Source: CAD feature listing. Evaluate the final solid. Frame: model axes, mm. A direction names the side the tool comes from. Coordinates: 2 decimals unless noted, no trailing zeros. Order: outer loops, then holes, each group sorted by start corner. A loop starts at its lowest first (then second) coordinate and runs counter-clockwise, first axis right, second up. Notation, with made-up numbers: (-37, 9.25) -> (21, 9.25) arc R34 cw to (21, 42.25) -> close; hole circle Ø8 at (6.25, 82.5). An arc over 180 degrees is marked (long way). Write item = value, one per line. Start each with the question number.
Item 1: Mould query, pull axis Z, two halves, no side actions, for faces 1 (the flat face through (-3.686, 11, 1)), 2 (the flat face through (27.7, -6.5, 36.367)), 3 (the flat face through (27, 10, 37)), 4 (the flat face through (-40, 10.642, 19)). Classes: released by +Z, released by -Z, zero draft, split by the parting line, or undercut.
Item 2: Ray query, line 1 along Y through (x, z) = (-41, 3); line 2 along Z through (x, y) = (-22, 14). Return the intervals inside material, ascending. Write a range as [from, to].
Item 3: Section query D-D (x = -39.5). Output: boundary loops of the cut face in (y, z).
Item 4: Section query B-B (z = 4.5). Output: boundary loops of the cut face in (x, y).
Item 5: Contact query for flat-ended pins moving along their axis: pin 1 (8 mm diameter, centred on x = -34.5, z = 12.5, fed in from -Y); pin 2 (1 mm diameter, centred on x = 28.5, z = 15.5, fed in from +Y); pin 3 (7.5 mm diameter, centred on y = -8.5, z = 12, fed in from -X). Output: stop coordinate, or through.
Item 6: Set-up query: faces 5 (the flat face through (29.47, -12, 20)), 6 (the flat face through (-38.216, -12, 20)), 7 (the flat face through (-41.716, 12, 20)), 8 (the flat face through (11, -13.208, 1)). Return all of +Z, -Z, +X, -X, +Y, -Y with unobstructed straight access to the full face (end or side cutting, diameter ignored); none if empty.
Item 7: Section query A-A (y = 0). Output: boundary loops of the cut face in (x, z).
Item 8: Section query C-C (x = 8). Output: boundary loops of the cut face in (y, z), then the cut area to 3 significant figures.
```python
from build123d import *

# Parameters (mm, degrees)
SKETCH1_W           = 105.78
SKETCH1_H           = 30
BOSS_EXTRUDE1_DEPTH = 2
SKETCH5_W           = 3.5
SKETCH5_H           = 2
BOSS_EXTRUDE2_DEPTH = 35
SKETCH6_W           = 3.5
SKETCH6_H           = 2
BOSS_EXTRUDE3_DEPTH = 35
SKETCH7_W           = 3.5
SKETCH7_H           = 0.495515405
BOSS_EXTRUDE4_DEPTH = 5
SKETCH9_W           = 3.5
SKETCH9_H           = 0.633233513
BOSS_EXTRUDE5_DEPTH = 5
SKETCH10_R          = 1.510168907
CUT_EXTRUDE2_DEPTH  = 72
SKETCH11_R          = 1.533572267
CUT_EXTRUDE3_DEPTH  = 42
SKETCH12_R          = 3.25
CUT_EXTRUDE4_DEPTH  = 15
FILLET1_R           = 0.8
SKETCH13_W          = 28.000104313
SKETCH13_H          = 4
CUT_EXTRUDE5_DEPTH  = 10


with BuildPart() as part:
    # Sketch1 → Boss-Extrude1 (new body)
    with BuildSketch(Plane.XY):
        Rectangle(SKETCH1_W, SKETCH1_H)
    extrude(amount=BOSS_EXTRUDE1_DEPTH)

    # Sketch5 → Boss-Extrude2 (add)
    with BuildSketch(Plane.XY.offset(2)):
        with Locations((27.719609025, 11.641851008)):
            Rectangle(SKETCH5_W, SKETCH5_H)
    boss_extrude2 = extrude(amount=BOSS_EXTRUDE2_DEPTH)

    # Sketch6 → Boss-Extrude3 (add)
    with BuildSketch(Plane.XY.offset(2)):
        with Locations((-39.966011677, 11.641851008)):
            Rectangle(SKETCH6_W, SKETCH6_H)
    boss_extrude3 = extrude(amount=BOSS_EXTRUDE3_DEPTH)

    # Sketch7 → Boss-Extrude4 (add)
    with BuildSketch(Plane.XZ.offset(-10.641851008)):
        with Locations((-39.966011677, 36.752242298)):
            Rectangle(SKETCH7_W, SKETCH7_H)
    boss_extrude4 = extrude(amount=BOSS_EXTRUDE4_DEPTH)

    # Sketch9 → Boss-Extrude5 (add)
    with BuildSketch(Plane.XZ.offset(-10.641851008)):
        with Locations((27.719609025, 36.683383244)):
            Rectangle(SKETCH9_W, SKETCH9_H)
    boss_extrude5 = extrude(amount=BOSS_EXTRUDE5_DEPTH)

    # Sketch10 → Cut-Extrude2 (cut)
    with BuildSketch(Plane.XY.offset(2)):
        with Locations(Location((27.719609025, 8.420134131, 0), (0, 0, 180))):
            Circle(SKETCH10_R)
    cut_extrude2 = extrude(amount=CUT_EXTRUDE2_DEPTH, mode=Mode.SUBTRACT)

    # Sketch11 → Cut-Extrude3 (cut)
    with BuildSketch(Plane.XY.offset(2)):
        with Locations(Location((-39.966011677, 8.661839338, 0), (0, 0, 180))):
            Circle(SKETCH11_R)
    cut_extrude3 = extrude(amount=CUT_EXTRUDE3_DEPTH, mode=Mode.SUBTRACT)

    # Mirror2: Boss-Extrude2, Boss-Extrude3, Boss-Extrude4, Boss-Extrude5, Cut-Extrude2, Cut-Extrude3 across plane
    add(boss_extrude2.mirror(Plane.ZX))
    add(boss_extrude3.mirror(Plane.ZX))
    add(boss_extrude4.mirror(Plane.ZX))
    add(boss_extrude5.mirror(Plane.ZX))
    add(cut_extrude2.mirror(Plane.ZX), mode=Mode.SUBTRACT)
    add(cut_extrude3.mirror(Plane.ZX), mode=Mode.SUBTRACT)

    # Sketch12 → Cut-Extrude4 (cut)
    with BuildSketch(Plane.XY.offset(2)):
        with Locations((-34.920285351, 0)):
            Circle(SKETCH12_R)
    extrude(amount=-CUT_EXTRUDE4_DEPTH, mode=Mode.SUBTRACT)

    # Fillet1
    fillet1_edges = [part.edges().sort_by_distance(p)[0] for p in [
        (29.469609025, 11.641851008, 2),
        (27.719609025, 12.641851008, 2),
        (25.969609025, 11.641851008, 2),
        (27.719609025, 10.641851008, 2),
        (-38.216011677, 11.641851008, 2),
        (-39.966011677, 12.641851008, 2),
        (-41.716011677, 11.641851008, 2),
        (-39.966011677, 10.641851008, 2),
        (29.469609025, -11.641851008, 2),
        (27.719609025, -12.641851008, 2),
        (25.969609025, -11.641851008, 2),
        (27.719609025, -10.641851008, 2),
        (-38.216011677, -11.641851008, 2),
        (-39.966011677, -12.641851008, 2),
        (-41.716011677, -11.641851008, 2),
        (-39.966011677, -10.641851008, 2),
    ]]
    fillet(fillet1_edges, radius=FILLET1_R)

    # Sketch13 → Cut-Extrude5 (cut)
    with BuildSketch(Plane(origin=(0, 0, 0), x_dir=(-1, 0, 0), z_dir=(0, 0, -1))):
        with Locations((-10.313745058, 11.208488392)):
            Rectangle(SKETCH13_W, SKETCH13_H)
    cut_extrude5 = extrude(amount=-CUT_EXTRUDE5_DEPTH, mode=Mode.SUBTRACT)

    # Mirror3: Cut-Extrude5 across plane
    add(cut_extrude5.mirror(Plane.ZX), mode=Mode.SUBTRACT)


solid = part.part
```
Computed:
q1.face_1 = zero draft
q1.face_2 = undercut
q1.face_3 = released by +Z
q1.face_4 = undercut
q2.line_1 = [-12.64, -10.64], [10.64, 12.64]
q2.line_2 = [0, 2]
q3.outline = (-15, 0) -> (15, 0) -> (15, 2) -> (13.44, 2) arc R0.8 cw to (12.64, 2.8) -> (12.64, 37) -> (10.12, 37) -> (10.12, 36.5) -> (10.64, 36.5) -> (10.64, 2.8) arc R0.8 cw to (9.84, 2) -> (-9.84, 2) arc R0.8 cw to (-10.64, 2.8) -> (-10.64, 36.5) -> (-10.12, 36.5) -> (-10.12, 37) -> (-12.64, 37) -> (-12.64, 2.8) arc R0.8 cw to (-13.44, 2) -> (-15, 2) -> close; (-7.2, 36.5) -> (-5.64, 36.5) -> (-5.64, 37) -> (-7.2, 37) -> close; (5.64, 36.5) -> (7.2, 36.5) -> (7.2, 37) -> (5.64, 37) -> close
q4.outline = (-41.72, -12.64) -> (-38.22, -12.64) -> (-38.22, -10.64) -> (-41.72, -10.64) -> close; (-41.72, 10.64) -> (-38.22, 10.64) -> (-38.22, 12.64) -> (-41.72, 12.64) -> close; (25.97, -12.64) -> (29.47, -12.64) -> (29.47, -10.64) -> (25.97, -10.64) -> close; (25.97, 10.64) -> (29.47, 10.64) -> (29.47, 12.64) -> (25.97, 12.64) -> close
q5.pin_1 = -12.64
q5.pin_2 = 12.64
q5.pin_3 = -41.72
q6.face_5 = +Z, +X, +Y, -Y
q6.face_6 = +Z, +Y, -Y
q6.face_7 = +Z, -X, +Y, -Y
q6.face_8 = +Z, -Z
q7.outline = (-52.89, 0) -> (-38.17, 0) -> (-38.17, 2) -> (-52.89, 2) -> close; (-31.67, 0) -> (52.89, 0) -> (52.89, 2) -> (-31.67, 2) -> close
q8.outline = (-15, 0) -> (-13.21, 0) -> (-13.21, 2) -> (-15, 2) -> close; (-9.21, 0) -> (9.21, 0) -> (9.21, 2) -> (-9.21, 2) -> close; (13.21, 0) -> (15, 0) -> (15, 2) -> (13.21, 2) -> close
q8.area = 44.0 mm^2
